Verification items for this drawing (mm, ordinates from the low corner). A direction names the side the tool comes from. Coordinates: 2 decimals unless noted, no trailing zeros. Loops run counter-clockwise (first coordinate to the right, second up) from the corner with the lowest first, then second, coordinate; pieces in that order, holes last. Notation, with made-up numbers: M 54.25,37 L 101.25,37 A24 ccw 101.25,76 Z; hole C 37.5,9 d2. An arc over 180 degrees is marked long. One line per question, with ' | ' between items. Start each with the question number.
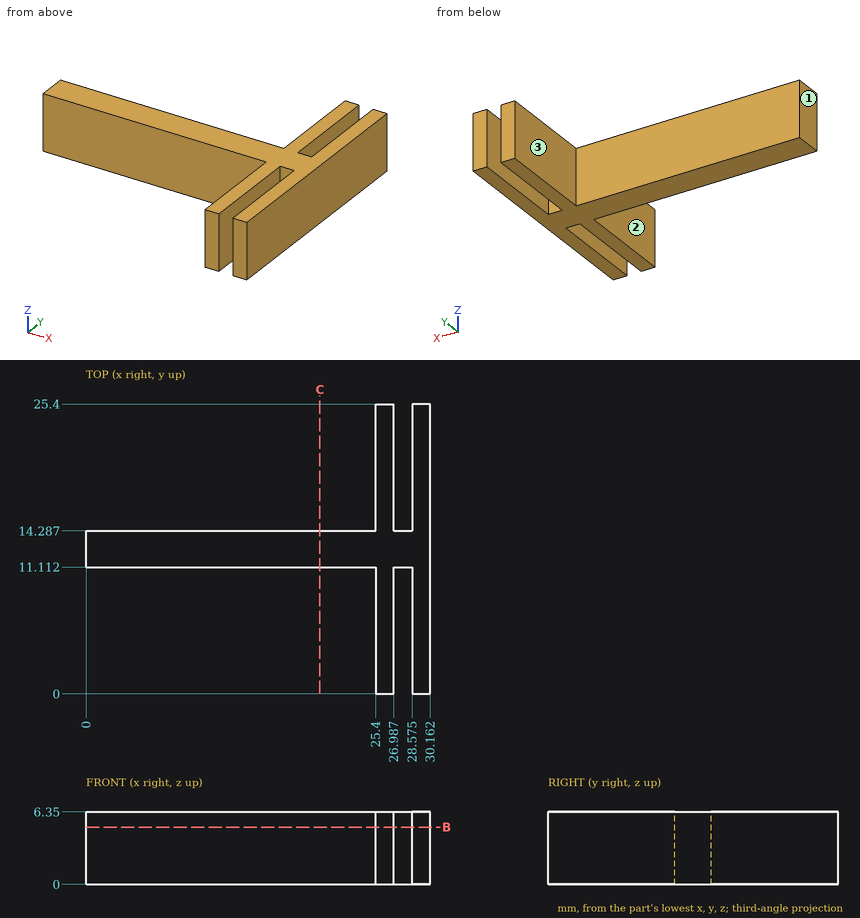
1. Thickness scan on line 1 (X direction, y = 10, z = 1.5) (1 decimal); line 2 (Y direction, x = 9, z = 1). Record the ranges inside material, lowest first.
2. Depth check by flat-ended pin: pin 1 Ø5 at (x, y) = (4.5, 7.5) entering from -Z; pin 2 Ø1.9 at (x, z) = (18, 3.5) entering from -Y; pin 3 Ø0.5 at (x, z) = (28, 1.5) entering from +Y; pin 4 Ø3 at (y, z) = (19, 3) entering from -X. Enter the tip coordinate at first touch or a pass-through.
3. Sectioned sample at B-B (z = 5). Record the cut outline in (x, y) (1 decimal), and give its area (3 significant figures).
4. Sectioned sample at C-C (x = 20.5). Record the cut outline in (y, z).
5. Tool access check on the marked faces 1, 2 and 3. Record the directions out of +Z, -Z, +X, -X, +Y, -Y that give a thin tool (end or side, any length) a straight path to the whole face; none if there is none.
Result:
1) line 1: x = 25.4 to 27, 28.6 to 30.2 | line 2: y = 11.11 to 14.29
2) pin 1: passes through | pin 2: stops at y = 11.11 | pin 3: stops at y = 14.29 | pin 4: stops at x = 25.4
3) outline: M 0,11.1 L 25.4,11.1 L 25.4,0 L 27,0 L 27,11.1 L 28.6,11.1 L 28.6,0 L 30.2,0 L 30.2,25.4 L 28.6,25.4 L 28.6,14.3 L 27,14.3 L 27,25.4 L 25.4,25.4 L 25.4,14.3 L 0,14.3 Z | area: 166 mm2
4) outline: M 11.11,0 L 14.29,0 L 14.29,6.35 L 11.11,6.35 Z
5) face 1: +Z, -Z, -X, +Y, -Y | face 2: +Z, -Z, -X, -Y | face 3: +Z, -Z, -X, +Y
